Could you check a few things on this model? Use its own coordinates, in mm. A direction names the side the tool comes from. Round coordinates to 2 decimals unless told otherwise and drop trailing zeros. Loops run counter-clockwise (first coordinate to the right, second up) from the corner with the lowest first, then second, coordinate; pieces in that order, holes last. Notation, with made-up numbers: M 12.25,68.25 L 40.25,68.25 A23 ccw 40.25,99.25 Z; hole C -8,1 d1. An arc over 180 degrees is marked long. One line per item, written item: value. Start each with the question number.
Q1. Imagine slicing it at A-A (x = -2.75). Please give me the cut outline in (y, z).
Q2. Thinking about a two-plate mould opening in Z: for faces 6 (the face through (-9, 5, 4)), 7 (the face through (-2, 5, -7)), 8 (the face through (-6, 10, -5)), 9 (the face through (-18.192, 4.93, 0.154)), which applies, released by +Z, released by -Z, zero draft, split by the parting line, or undercut?
Q3. I'm going to push flat-ended pins straight in: pin 1 Ø0.6 at (y, z) = (5.5, -5.5) entering from -X; pin 2 Ø1.1 at (y, z) = (6.5, 5.5) entering from -X; pin 3 Ø1 at (y, z) = (6.5, -0.5) entering from -X; pin 4 Ø1.2 at (y, z) = (6.5, 4.5) entering from +X. Where does each tip first touch, or does it pass through?
Q4. Imagine slicing it at D-D (y = 7). Give the number of separate pieces and of enclosed holes in the cut face, then the cut area to 3 significant figures.
Q5. Imagine slicing it at B-B (y = 9.5). Please give me the cut outline in (x, z), then the cut area to 3 significant figures.
Q6. Please list where these lines run through material, in increasing order: line 1 along Y through (x, z) = (5, -4); line 2 along X through (y, z) = (7.25, -6); line 3 along X through (y, z) = (3, 1.25).
Q7. Imagine slicing it at C-C (z = 0). Please give me the cut outline in (x, y), then the cut area to 3 significant figures.
Q8. Which directions (+Z, -Z, +X, -X, +Y, -Y) give clear straight access to the entire face, cutting with the end or side of a thin tool? Please do faces 1 (the face through (3.94, 7.07, 5.5)), 2 (the face through (-3, 5, 4)), 3 (the face through (4, 3, -6)), 4 (the face through (-4, 5, 7)), 5 (the face through (7, 5, 0)).
Autodesk Inventor part; units mm, degrees
ref_plane "YZ Plane" through (0, 0, 0) normal (1, 0, 0) x (0, 1, 0)
ref_plane "XZ Plane" through (0, 0, 0) normal (0, 1, 0) x (-1, 0, 0)
ref_plane "XY Plane" through (0, 0, 0) normal (0, 0, 1) x (1, 0, 0)
sketch "Sketch1" plane through (0, 0, 0) normal (0, 1, 0) x (-1, 0, 0)
  arc A0 (0, 4) -> (0, -4) centre (0, 0) ccw
  arc A1 (11.1938, -4) -> (11.1938, 4) centre (11.1938, 0) ccw
  line L0 (11.1938, -4) -> (0, -4)
  line L1 (11.1938, 4) -> (0, 4)
  line L2 (11.1938, -7) -> (0, -7)
  line L3 (0, 7) -> (11.1938, 7)
  arc A2 (5.5969, 4.2041) -> (5.4492, 4) centre (11.1938, 0) ccw
  arc A3 (5.7446, 4) -> (5.5969, 4.2041) centre (0, 0) ccw
  arc A4 (5.4492, -4) -> (5.5969, -4.2041) centre (11.1938, 0) ccw
  arc A5 (11.1938, -7) -> (11.1938, 7) centre (11.1938, 0) ccw
  arc A6 (0, 7) -> (0, -7) centre (0, 0) ccw
  arc A7 (5.5969, -4.2041) -> (5.7446, -4) centre (0, 0) ccw
  dimension "d0" = 8
  dimension "d1" = 8
extrude "Extrusion1" add sketch "Sketch1" along normal blind 10
sketch "Sketch2" plane through (0, 0, 0) normal (0, -1, 0) x (1, 0, 0)
  arc A0 (0, -7) -> (0, 7) centre (0, 0) ccw
  arc A1 (0, -4) -> (0, 4) centre (0, 0) ccw
  line L0 (0, -7) -> (0, -4)
  line L1 (0, 4) -> (0, 7)
  line L2 (0, -7) -> (-11.1938, -7)
  line L3 (0, -7) -> (5, -7)
  arc A2 (0, -7) -> (0, 7) centre (0, 0) ccw
  line L4 (0, 7) -> (5, 7)
  line L5 (5, 7) -> (5, -7)
  dimension "d6" = 5
extrude "Extrusion2" add sketch "Sketch2" against normal blind 3 contours L0 A1 L1 A0 L5 | A0 L5 L3 | A0 L4 L5
sketch "Sketch3" plane through (5, 0, 7) normal (1, 0, 0) x (0, 0, -1)
  line L0 (14, 10) -> (0, 10)
  line L1 (0, 0) -> (14, 0)
  line L2 (14, 0) -> (14, 10)
  line L3 (14, 10) -> (0, 10)
  line L4 (0, 10) -> (0, 0)
  point P0 (7, 0)
extrude "Extrusion3" add sketch "Sketch3" along normal blind 2
sketch "Sketch4" plane through (7, 0, 7) normal (1, 0, 0) x (0, 0, -1)
  circle A0 centre (3, 7) radius 1.5
  circle A1 centre (11, 7) radius 1.5
  line L0 (14, 10) -> (0, 10)
  line L1 (0, 10) -> (0, 0)
  line L2 (14, 0) -> (14, 10)
  point P0 (7, 0)
  dimension "d11" = 3
  dimension "d12" = 3
  dimension "d13" = 3
  dimension "d14" = 3
  dimension "d15" = 3
  dimension "d16" = 3
extrude "Extrusion4" cut sketch "Sketch4" against normal blind 8
sketch "Sketch5" plane through (0, 10, 0) normal (0, 1, 0) x (1, 0, 0)
  point P0 (0, 0)
sketch "Sketch6" plane through (0, 10, 0) normal (0, 1, 0) x (1, 0, 0)
  point P0 (0, 0)
properties part number "bedtiedown3"
Report:
1. outline: M 0,-7 L 10,-7 L 10,-4 L 0,-4 Z; M 0,4 L 10,4 L 10,7 L 0,7 Z
2. face 6: undercut
2. face 7: released by -Z
2. face 8: zero draft
2. face 9: split by the parting line
3. pin 1: stops at x = -15.88
3. pin 2: stops at x = -16.14
3. pin 3: stops at x = -18.19
3. pin 4: stops at x = -1
4. separate pieces: 4
4. enclosed holes: 0
4. area: 147 mm²
5. outline: M -11.19,-7 L 0,-7 A7 ccw 5,-4.9 L 5,-7 L 7,-7 L 7,7 L 5,7 L 5,4.9 A7 ccw 0,7 L -11.19,7 A7 ccw Z; hole M -11.19,-4 L -5.74,-4 A7.15 ccw -5.6,-4.2 A6.85 ccw -5.45,-4 L 0,-4 A4 ccw 0,4 L -5.45,4 A7.15 ccw -5.6,4.2 A6.85 ccw -5.74,4 L -11.19,4 A4 ccw Z
5. area: 185 mm²
6. line 1: y = 0 to 5.5, 8.5 to 10
6. line 2: x = -14.8 to 3.61, 5 to 7
6. line 3: x = -18.08 to -14.99, 3.8 to 7
7. outline: M -18.19,0 L -15.19,0 L -15.19,10 L -18.19,10 Z; M 4,0 L 7,0 L 7,10 L 4,10 Z
7. area: 60.0 mm²
8. face 1: +X
8. face 2: +Y, -Y
8. face 3: -Z, +Y
8. face 4: +Z, +X, -X, +Y, -Y
8. face 5: +Z, -Z, +X, +Y, -Y
